Part model, mm, in its own coordinate system. A direction names the side the tool comes from. Round coordinates to 2 decimals unless told otherwise and drop trailing zeros. Write each loop counter-clockwise with the first axis right and the second up, starting at its lowest first coordinate (ties: lowest second). Pieces come first, ordered by that corner, then holes.
Autodesk Inventor part; units mm, degrees
ref_plane "YZ Plane" through (0, 0, 0) normal (1, 0, 0) x (0, 1, 0)
ref_plane "XZ Plane" through (0, 0, 0) normal (0, 1, 0) x (-1, 0, 0)
ref_plane "XY Plane" through (0, 0, 0) normal (0, 0, 1) x (1, 0, 0)
sketch "Sketch1" plane through (0, 0, 0) normal (0, 0, 1) x (1, 0, 0)
  line L0 (-11, 43) -> (11, 43)
  line L1 (11, 43) -> (11, -43)
  line L2 (11, -43) -> (-11, -43)
  line L3 (-11, -43) -> (-11, 43)
  line L4 (-11, 43) -> (11, -43) construction
  line L5 (11, 43) -> (-11, -43) construction
  circle A0 centre (-8, 40.5) radius 1
  circle A1 centre (8, 40.5) radius 1
  circle A2 centre (-8, -40.5) radius 1
  circle A3 centre (8, -40.5) radius 1
  line L6 (7, 38) -> (-7, 38)
  line L7 (-7, 38) -> (-7, -38)
  line L8 (-7, -38) -> (7, -38)
  line L9 (7, -38) -> (7, 38)
  line L10 (7, 38) -> (-7, -38) construction
  line L11 (-7, 38) -> (7, -38) construction
  point P0 (0, 0)
  dimension "d0" = 22
  dimension "d1" = 86
  dimension "d2" = 2
  dimension "d3" = 2
  dimension "d4" = 2
  dimension "d5" = 2
  dimension "d6" = 3
  dimension "d7" = 2.5
  dimension "d8" = 3
  dimension "d9" = 2.5
  dimension "d10" = 2.5
  dimension "d11" = 3
  dimension "d12" = 3
  dimension "d13" = 2.5
  dimension "d14" = 14
  dimension "d15" = 76
extrude "Extrusion1" add sketch "Sketch1" along normal blind 4
properties part number "PartC_3D"
Q1. Cut at B-B on y = -40.5. Write the cut outline in (x, z).
Values follow:
outline: (-11, 0) - (-9, 0) - (-9, 4) - (-11, 4) - close; (-7, 0) - (7, 0) - (7, 4) - (-7, 4) - close; (9, 0) - (11, 0) - (11, 4) - (9, 4) - close
Q2. Wall check: L1, parallel to Y at x = -8, z = 1.5; L2, parallel to X at y = 2.5, z = 3.1; L3, parallel to Y at x = -0.25, z = 2.25. Give the ranges that are in metal, low to high.
Values follow:
L1: y = -43 to -41.5, -39.5 to 39.5, 41.5 to 43
L2: x = -11 to -7, 7 to 11
L3: y = -43 to -38, 38 to 43
Q3. Which spindle directions (+Z, -Z, +X, -X, +Y, -Y) get a long thin tool onto all of the face, cutting with end or side? Do faces 5 (the flat face through (11, 1, 2)), 6 (the flat face through (7, -1, 2)). Say none if no direction does.
Values follow:
face 5: +Z, -Z, +X, +Y, -Y
face 6: +Z, -Z
Q4. Cut at D-D on x = -8. Write the cut outline in (y, z).
Values follow:
outline: (-43, 0) - (-41.5, 0) - (-41.5, 4) - (-43, 4) - close; (-39.5, 0) - (39.5, 0) - (39.5, 4) - (-39.5, 4) - close; (41.5, 0) - (43, 0) - (43, 4) - (41.5, 4) - close
Q5. Mould opens along X. For faces 1 (the cylindrical face through (-8.13, 39.51, 1.97)), 2 (the cylindrical face through (7.87, 39.51, 1.97)), 3 (the flat face through (-7.5, 0.6, 0)), 4 (the flat face through (-11, -1, 2)) say: +X half, -X half, draft (parallel to the pull), parting line (faces both ways), or undercut.
Values follow:
face 1: undercut
face 2: undercut
face 3: draft
face 4: -X half
Q6. Cut at C-C on y = 36. Write the cut outline in (x, z).
Values follow:
outline: (-11, 0) - (-7, 0) - (-7, 4) - (-11, 4) - close; (7, 0) - (11, 0) - (11, 4) - (7, 4) - close
Q7. Cut at A-A on x = 0.25. Write the cut outline in (y, z).
Values follow:
outline: (-43, 0) - (-38, 0) - (-38, 4) - (-43, 4) - close; (38, 0) - (43, 0) - (43, 4) - (38, 4) - close
